Here's how the part is built. I have some questions about the finished solid (model axes, mm). Face numbers are marked on the shaded views. A direction names the side the tool comes from. Give positions to 0.01 mm unless a question says otherwise; leave off trailing zeros. Order: outer loops, then holes, each group sorted by start corner. A loop starts at its lowest first (then second) coordinate and runs counter-clockwise, first axis right, second up. Notation, with made-up numbers: (-36.75, -24) -> (-13.75, -24) arc R30 ccw to (-13.75, -1) -> close; hole circle Ø10 at (71.25, 72.25). An arc over 180 degrees is marked (long way). Write each question's results on one line, items separated by ' | '. Start each with the question number.
Q1. Thinking about a two-plate mould opening in Y: for the marked faces 1, 2 and 3, which applies, pulls with the +Y half, pulls with the -Y half, needs draft (parallel to the pull), parting line crosses it, or undercut?
Q2. Imagine slicing it at C-C, the plane y = -18.5. Please give me the cut outline in (x, z).
Q3. I need wall thicknesses on line 1 along Y through (x, z) = (4.4, -15); line 2 along Z through (x, y) = (0, 23); line 3 along X through (y, z) = (21, -11.5). Which ranges of each line are inside material? Lowest first, please. Write a range as [from, to].
Q4. Imagine slicing it at D-D, the plane z = -9.5. Please give me the cut outline in (x, y).
Q5. Imagine slicing it at B-B, the plane x = 0. Please give me the cut outline in (y, z).
Q6. I'm going to push flat-ended pins straight in: pin 1 (2.5 mm diameter, centred on y = -23.5, z = 1, fed in from -X); pin 2 (8 mm diameter, centred on x = -19, z = -5, fed in from +Y); pin 3 (0.9 mm diameter, centred on y = -16, z = 1.5, fed in from -X); pin 4 (5 mm diameter, centred on x = -16, z = -10.5, fed in from -Y). Where does each tip first touch, or does it pass through?
Q7. Imagine slicing it at A-A, the plane z = -15. Please give me the cut outline in (x, y).
Q8. For the marked faces 4, 5 and 6, which set-ups out of +Z, -Z, +X, -X, +Y, -Y let a thin tool reach every point of the face, with its end or its side?
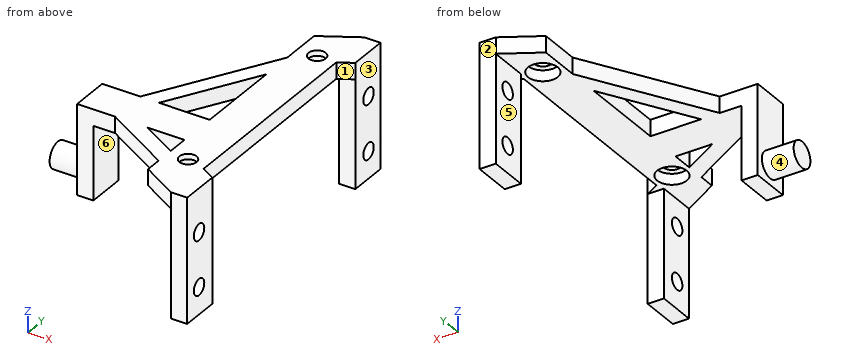
```python
from build123d import *

# Parameters (mm, degrees)
SKETCH1_R           = 1.6
BOSS_EXTRUDE1_DEPTH = 3
SKETCH2_R           = 2.75
CUT_EXTRUDE1_DEPTH  = 2
SKETCH4_W           = 3
SKETCH4_H           = 7.2
BOSS_EXTRUDE2_DEPTH = 20
CUT_EXTRUDE2_REACH  = 5.01
SKETCH5_R           = 1.4975
SKETCH7_W           = 13.6
SKETCH7_H           = 7.2
BOSS_EXTRUDE3_DEPTH = 3
SKETCH8_R           = 2.4
BOSS_EXTRUDE4_DEPTH = 5.89


with BuildPart() as part:
    # Sketch1 → Boss-Extrude1 (new body)
    with BuildSketch(Plane.XY):
        Polygon((3.6, 18.431983311), (3.6, -19.596209808), (6.17, -21.08), (6.17, -28.28), (3.17, -28.28), (-3.6, -24.371338678), (-3.6, -21.371338678), (-16.45413565, -13.95), (-20.5, -13.95), (-23.5, -13.95), (-23.5, -6.75), (-20.5, -6.75), (-16.45413565, -6.75), (-3.6, 15.514016033), (-3.6, 23.20711218), (3.16, 27.11), (6.16, 27.11), (6.16, 19.91), align=None)
        with Locations((0, 18.5)):
            Circle(SKETCH1_R, mode=Mode.SUBTRACT)
        with Locations((0, -18.5)):
            Circle(SKETCH1_R, mode=Mode.SUBTRACT)
        Polygon((-10.45413565, -13.95), (-3.6, -13.95), (-3.6, -17.907237062), align=None, mode=Mode.SUBTRACT)
        Polygon((-3.6, -6.75), (-12.990034035, -6.75), (-3.6, 9.514016033), align=None, mode=Mode.SUBTRACT)
    extrude(amount=BOSS_EXTRUDE1_DEPTH)

    # Sketch2 → Cut-Extrude1 (cut)
    with BuildSketch(Plane(origin=(0, 0, 0), x_dir=(-1, 0, 0), z_dir=(0, 0, -1))):
        with Locations((0, 18.5)):
            Circle(SKETCH2_R)
        with Locations((0, -18.5)):
            Circle(SKETCH2_R)
    extrude(amount=-CUT_EXTRUDE1_DEPTH, mode=Mode.SUBTRACT)

    # Sketch4 → Boss-Extrude2 (add)
    with BuildSketch(Plane(origin=(0, 0, 0), x_dir=(-1, 0, 0), z_dir=(0, 0, -1))):
        with Locations((-4.66, 23.51)):
            Rectangle(SKETCH4_W, SKETCH4_H)
        with Locations((-4.67, -24.68)):
            Rectangle(SKETCH4_W, SKETCH4_H)
    extrude(amount=BOSS_EXTRUDE2_DEPTH)

    # Sketch5 → Cut-Extrude2 (cut, up to next)
    with BuildSketch(Plane.ZY.offset(-3.16), mode=Mode.PRIVATE) as cut_extrude2_sk1:
        with Locations((-5, 23.71)):
            Circle(SKETCH5_R)
    cut_extrude2_tool1 = extrude(cut_extrude2_sk1.sketch, amount=-CUT_EXTRUDE2_REACH, mode=Mode.PRIVATE) & part.part
    add(cut_extrude2_tool1.solids().sort_by_distance((3.16, 23.71, -5))[0], mode=Mode.SUBTRACT)
    # Sketch5 → Cut-Extrude2 (cut, up to next)
    with BuildSketch(Plane.ZY.offset(-3.16), mode=Mode.PRIVATE) as cut_extrude2_sk2:
        with Locations((-15, 23.71)):
            Circle(SKETCH5_R)
    cut_extrude2_tool2 = extrude(cut_extrude2_sk2.sketch, amount=-CUT_EXTRUDE2_REACH, mode=Mode.PRIVATE) & part.part
    add(cut_extrude2_tool2.solids().sort_by_distance((3.16, 23.71, -15))[0], mode=Mode.SUBTRACT)
    # Sketch5 → Cut-Extrude2 (cut, up to next)
    with BuildSketch(Plane.ZY.offset(-3.16), mode=Mode.PRIVATE) as cut_extrude2_sk3:
        with Locations((-15, -24.88)):
            Circle(SKETCH5_R)
    cut_extrude2_tool3 = extrude(cut_extrude2_sk3.sketch, amount=-CUT_EXTRUDE2_REACH, mode=Mode.PRIVATE) & part.part
    add(cut_extrude2_tool3.solids().sort_by_distance((3.16, -24.88, -15))[0], mode=Mode.SUBTRACT)
    # Sketch5 → Cut-Extrude2 (cut, up to next)
    with BuildSketch(Plane.ZY.offset(-3.16), mode=Mode.PRIVATE) as cut_extrude2_sk4:
        with Locations((-5, -24.88)):
            Circle(SKETCH5_R)
    cut_extrude2_tool4 = extrude(cut_extrude2_sk4.sketch, amount=-CUT_EXTRUDE2_REACH, mode=Mode.PRIVATE) & part.part
    add(cut_extrude2_tool4.solids().sort_by_distance((3.16, -24.88, -5))[0], mode=Mode.SUBTRACT)

    # Sketch7 → Boss-Extrude3 (add)
    with BuildSketch(Plane.ZY.offset(23.5)):
        with Locations((-6.8, -10.35)):
            Rectangle(SKETCH7_W, SKETCH7_H)
    extrude(amount=-BOSS_EXTRUDE3_DEPTH)

    # Sketch8 → Boss-Extrude4 (add)
    with BuildSketch(Plane.ZY.offset(23.5)):
        with Locations((-10, -10.35)):
            Circle(SKETCH8_R)
    extrude(amount=BOSS_EXTRUDE4_DEPTH)


solid = part.part
```
Geometry check:
1) face 1: undercut | face 2: pulls with the +Y half | face 3: needs draft
2) outline: (-8.57, 0) -> (-2.75, 0) -> (-2.75, 2) -> (-1.6, 2) -> (-1.6, 3) -> (-8.57, 3) -> close; (1.6, 2) -> (2.75, 2) -> (2.75, 0) -> (3.6, 0) -> (3.6, 3) -> (1.6, 3) -> close
3) line 1: [-28.28, -26.38], [-23.38, -21.08], [19.91, 22.21], [25.21, 27.11] | line 2: [0, 3] | line 3: [3.16, 6.16]
4) outline: (-29.39, -12.7) -> (-23.5, -12.7) -> (-23.5, -13.95) -> (-20.5, -13.95) -> (-20.5, -6.75) -> (-23.5, -6.75) -> (-23.5, -8) -> (-29.39, -8) -> close; (3.16, 19.91) -> (6.16, 19.91) -> (6.16, 27.11) -> (3.16, 27.11) -> close; (3.17, -28.28) -> (6.17, -28.28) -> (6.17, -21.08) -> (3.17, -21.08) -> close
5) outline: (-26.45, 0) -> (-21.25, 0) -> (-21.25, 2) -> (-20.1, 2) -> (-20.1, 3) -> (-26.45, 3) -> close; (-16.9, 2) -> (-15.75, 2) -> (-15.75, 0) -> (15.75, 0) -> (15.75, 2) -> (16.9, 2) -> (16.9, 3) -> (-16.9, 3) -> close; (20.1, 2) -> (21.25, 2) -> (21.25, 0) -> (25.29, 0) -> (25.29, 3) -> (20.1, 3) -> close
6) pin 1: x = -3.6 | pin 2: y = -6.75 | pin 3: x = -13.68 | pin 4: through
7) outline: (3.16, 19.91) -> (6.16, 19.91) -> (6.16, 22.21) -> (3.16, 22.21) -> close; (3.16, 25.21) -> (6.16, 25.21) -> (6.16, 27.11) -> (3.16, 27.11) -> close; (3.17, -28.28) -> (6.17, -28.28) -> (6.17, -26.38) -> (3.17, -26.38) -> close; (3.17, -23.38) -> (6.17, -23.38) -> (6.17, -21.08) -> (3.17, -21.08) -> close
8) face 4: -X | face 5: -Z, -X, +Y, -Y | face 6: -Z, +X, +Y, -Y
